from build123d import *

# Parameters (mm, degrees)
EXTRUDE_1_DEPTH      = 30
SKETCH_2_R           = 1.25
CUT_EXTRUDE_1_DEPTH  = 58.306195128
SKETCH_4_W           = 4
SKETCH_4_H           = 24
CUT_EXTRUDE_2_DEPTH  = 4.5
SKETCH_5_R           = 1.75
CUT_EXTRUDE_3_DEPTH  = 61.166435826
EXTRUDE_2_DEPTH      = 2
EXTRUDE_2_DEPTH_BACK = 2


with BuildPart() as part:
    # Эскиз1 → Бобышка-Вытянуть1 (new body)
    with BuildSketch(Plane.XY):
        Polygon((0, 0), (0, 24), (-40, 24), (-40, 28), (4, 28), (4, 0), align=None)
    extrude(amount=-EXTRUDE_1_DEPTH)

    # Эскиз2 → Вырез-Вытянуть1 (cut, through all)
    with BuildSketch(Plane(origin=(0, 28, 0), x_dir=(1, 0, 0), z_dir=(0, 1, 0))):
        with Locations(Location((-37, 3, 0), (0, 0, 270))):
            Circle(SKETCH_2_R)
        with Locations(Location((-13, 3, 0), (0, 0, 270))):
            Circle(SKETCH_2_R)
        with Locations(Location((-37, 27, 0), (0, 0, 270))):
            Circle(SKETCH_2_R)
        with Locations(Location((-37, 15, 0), (0, 0, 270))):
            Circle(SKETCH_2_R)
        with Locations(Location((-25, 27, 0), (0, 0, 270))):
            Circle(SKETCH_2_R)
        with Locations(Location((-13, 27, 0), (0, 0, 270))):
            Circle(SKETCH_2_R)
        with Locations(Location((-13, 15, 0), (0, 0, 270))):
            Circle(SKETCH_2_R)
        with Locations(Location((-25, 3, 0), (0, 0, 270))):
            Circle(SKETCH_2_R)
        with Locations(Location((-25, 15, 0), (0, 0, 270))):
            Circle(SKETCH_2_R)
    extrude(amount=-CUT_EXTRUDE_1_DEPTH, mode=Mode.SUBTRACT)

    # Эскиз4 → Вырез-Вытянуть2 (cut)
    with BuildSketch(Plane.XY):
        with Locations((2, 12)):
            Rectangle(SKETCH_4_W, SKETCH_4_H)
    cut_extrude_2 = extrude(amount=-CUT_EXTRUDE_2_DEPTH, mode=Mode.SUBTRACT)

    # Зеркальное отражение1: Вырез-Вытянуть2 across plane
    add(cut_extrude_2.mirror(Plane.XY.offset(-15)), mode=Mode.SUBTRACT)

    # Эскиз5 → Вырез-Вытянуть3 (cut, through all)
    with BuildSketch(Plane(origin=(4, 0, 0), x_dir=(0, 0, -1), z_dir=(1, 0, 0))):
        with Locations(Location((9, 19, 0), (0, 0, 90))):
            Circle(SKETCH_5_R)
        with Locations(Location((21, 19, 0), (0, 0, 90))):
            Circle(SKETCH_5_R)
        with Locations(Location((21, 8, 0), (0, 0, 90))):
            Circle(SKETCH_5_R)
        with Locations(Location((9, 8, 0), (0, 0, 90))):
            Circle(SKETCH_5_R)
    extrude(amount=-CUT_EXTRUDE_3_DEPTH, mode=Mode.SUBTRACT)

    # Эскиз8 → Бобышка-Вытянуть2 (add, two sides: drawn at the far end of the back side and taken through both)
    with BuildSketch(Plane.XY.offset(-15).offset(-EXTRUDE_2_DEPTH_BACK)):
        Polygon((0, 0), (0, 24), (-8, 24), align=None)
    extrude(amount=EXTRUDE_2_DEPTH + EXTRUDE_2_DEPTH_BACK)


solid = part.part
Verification items for the finished model (mm, model axes). A direction names the side the tool comes from. Coordinates: 2 decimals unless noted, no trailing zeros. Loops run counter-clockwise (first coordinate to the right, second up) from the corner with the lowest first, then second, coordinate; pieces in that order, holes last. Notation, with made-up numbers: M 3.25,1 L 12.25,1 A12 cw 12.25,16 Z; hole C 87,47.5 d2. An arc over 180 degrees is marked long. One line per item, written item: value.
1. Section check C-C on y = 5.25. Record the cut outline in (x, z), plus the area to 3 significant figures.
Answers follow:
outline: M -1.75,-17 L 0,-17 L 0,-25.5 L 4,-25.5 L 4,-4.5 L 0,-4.5 L 0,-13 L -1.75,-13 Z
area: 91.0 mm^2
2. Section check A-A on x = -37. Record the cut outline in (y, z).
Answers follow:
outline: M 24,-30 L 28,-30 L 28,-28.25 L 24,-28.25 Z; M 24,-25.75 L 28,-25.75 L 28,-16.25 L 24,-16.25 Z; M 24,-13.75 L 28,-13.75 L 28,-4.25 L 24,-4.25 Z; M 24,-1.75 L 28,-1.75 L 28,0 L 24,0 Z
3. Section check B-B on z = -27. Record the cut outline in (x, y).
Answers follow:
outline: M -40,24 L -38.25,24 L -38.25,28 L -40,28 Z; M -35.75,24 L -26.25,24 L -26.25,28 L -35.75,28 Z; M -23.75,24 L -14.25,24 L -14.25,28 L -23.75,28 Z; M -11.75,24 L 4,24 L 4,28 L -11.75,28 Z
4. Material ranges on line 1 along X through (y, z) = (25.35, -15); line 2 along Z through (x, y) = (2.65, 8); line 3 along Y through (x, z) = (1, -8.5), recorded low to high. Write a range as from..to.
Answers follow:
line 1: -40..-38.25, -35.75..-26.25, -23.75..-14.25, -11.75..4
line 2: -25.5..-22.75, -19.25..-10.75, -7.25..-4.5
line 3: 0..6.32, 9.68..17.32, 20.68..28
5. Section check D-D on y = 19. Record the cut outline in (x, z), plus the area to 3 significant figures.
Answers follow:
outline: M -6.33,-17 L 0,-17 L 0,-19.25 L 4,-19.25 L 4,-10.75 L 0,-10.75 L 0,-13 L -6.33,-13 Z; M 0,-25.5 L 4,-25.5 L 4,-22.75 L 0,-22.75 Z; M 0,-7.25 L 4,-7.25 L 4,-4.5 L 0,-4.5 Z
area: 81.3 mm^2
6. Mould release check, pull along X, two halves, no side actions. Record for faces 4 (the flat face through (-18, 24, -15)), 5 (the flat face through (0, 12, -9)), 6 (the cylindrical face through (-11.946, 26.028, -2.328)): pulls with the +X half, pulls with the -X half, needs draft (parallel to the pull), parting line crosses it, or undercut.
Answers follow:
face 4: needs draft
face 5: pulls with the -X half
face 6: undercut
7. Set-up check for faces 1 (the flat face through (2, 12, -25.5)), 2 (the flat face through (2, 12, -4.5)), 3 (the flat face through (-2, 18, -17)): record each of +Z, -Z, +X, -X, +Y, -Y from which the full face is reachable in a straight line by a thin tool's end or side.
Answers follow:
face 1: -Z, +X, -X, -Y
face 2: +Z, +X, -X, -Y
face 3: -Z, -X, -Y
8. Gauge pin test, flat ends, axial feed: P1, Ø3, axis at x = -37, z = -27, coming from the -Y side; P2, Ø3, axis at x = -7.5, y = 17.5, coming from the -Z side; P3, Ø4, axis at x = -37, z = -3, coming from the +Y side; P4, Ø1, axis at y = 21.5, z = -11.5, coming from the -X side. Record the tip position at first contact, or that the pin passes through.
Answers follow:
P1: y = 24
P2: through
P3: y = 28
P4: x = 0
